Part print with two shaded views. Sizes in mm from the minimum x, y, z corner. A direction names the side the tool comes from. Coordinates: 2 decimals unless noted, no trailing zeros. Loops run counter-clockwise (first coordinate to the right, second up) from the corner with the lowest first, then second, coordinate; pieces in that order, holes last.
Item 1: Flat gauge pin, fed straight in: pin 1 (1 mm diameter, centred on x = 10.5, z = 1, fed in from +Y). Where does the tip first touch, or does it go through?
Item 2: Drill centre lines: line 1 along Y through (x, z) = (6.8, 4.75); line 2 along Y through (x, z) = (6.8, 1.35); line 3 along Z through (x, y) = (2.25, 9.25). Where is each one in solid material? Low to high.
Item 3: Cut at D-D (y = 1.5). List the corners of the cut face in (x, z), and give its area (3 significant figures).
Item 4: Cut at B-B (z = 1.6). List the corners of the cut face in (x, y) (3 decimals), and give its area (3 significant figures).
Item 5: Cut at A-A (x = 6.8). List the corners of the cut face in (y, z).
Item 6: Cut at C-C (x = 9.5). List the corners of the cut face in (y, z).
Item 7: 3-axis set-ups, long thin cutter, end or side, ignore diameter. For the marked faces 1 and 2: which of +Z, -Z, +X, -X, +Y, -Y reach the whole face in a straight line?
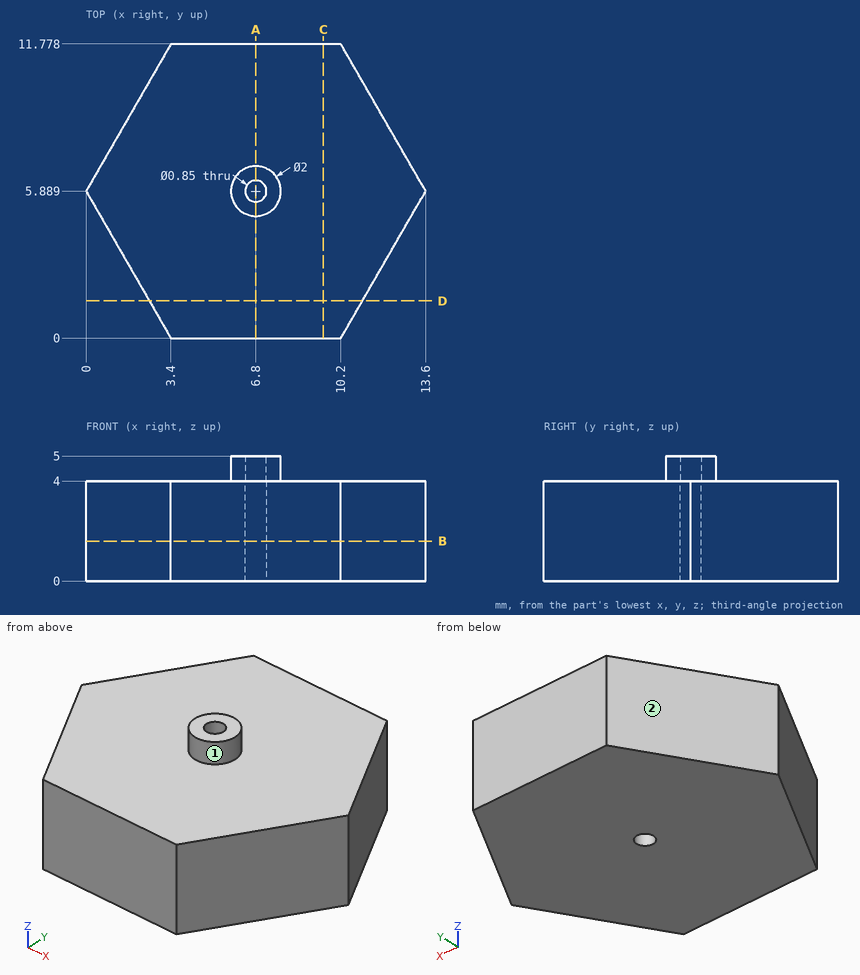
Filled sheet:
1. pin 1: stops at y = 11.78
2. line 1: y = 4.89 to 5.46, 6.31 to 6.89
2. line 2: y = 0 to 5.46, 6.31 to 11.78
2. line 3: z = 0 to 4
3. outline: (2.53, 0) - (11.07, 0) - (11.07, 4) - (2.53, 4) - close
3. area: 34.1 mm2
4. outline: (0, 5.889) - (3.4, 0) - (10.2, 0) - (13.6, 5.889) - (10.2, 11.778) - (3.4, 11.778) - close; hole circle Ø0.85 at (6.8, 5.889)
4. area: 120 mm2
5. outline: (0, 0) - (5.46, 0) - (5.46, 5) - (4.89, 5) - (4.89, 4) - (0, 4) - close; (6.31, 0) - (11.78, 0) - (11.78, 4) - (6.89, 4) - (6.89, 5) - (6.31, 5) - close
6. outline: (0, 0) - (11.78, 0) - (11.78, 4) - (0, 4) - close
7. face 1: +Z
7. face 2: +Z, -Z, -X, +Y
